Input: dimensioned drawing with shaded views. Units: mm. Origin: part minimum x, y, z. A direction names the side the tool comes from. Coordinates: 2 decimals unless noted, no trailing zeros. Write each loop counter-clockwise with the first axis right and the second up, starting at its lowest first coordinate (ties: lowest second). Pieces come first, ordered by that corner, then holes. Notation, with made-up numbers: (14, 38.5) -> (72, 38.5) arc R26 ccw to (72, 60.5) -> close; hole circle Ø5 at (26.5, 65). An arc over 180 degrees is marked (long way). One line per item, written item: value. Start each with the question number.
1. Section query B-B, the plane y = 13. Output: boundary loops of the cut face in (x, z) (1 decimal).
2. Access query for the marked faces 3 and 4. Directions: +Z, -Z, +X, -X, +Y, -Y. A direction counts if a zero-diameter tool reaches every point of the face in a straight line with its end or side. Return the directions, or none.
3. Line query: line 1 (Y direction, x = 0.95, z = 12.5); line 2 (Y direction, x = 0.25, z = 3.5) (1 decimal); line 3 (Z direction, x = 0.35, y = 10.5) (1 decimal). Output: solid intervals per line, ascending.
4. Section query D-D, the plane z = 7.75. Output: boundary loops of the cut face in (x, y).
5. Section query C-C, the plane y = 8.5. Output: boundary loops of the cut face in (x, z) (1 decimal).
6. First-contact query: P1, Ø0.5, axis at x = 0.5, y = 15.5, coming from the +Z side. Flat tip, straight axial feed; report the tip coordinate or a pass-through.
7. Mould query, pull axis Z, two halves, no side actions, for the marked faces 1 and 2. Classes: released by +Z, released by -Z, zero draft, split by the parting line, or undercut.
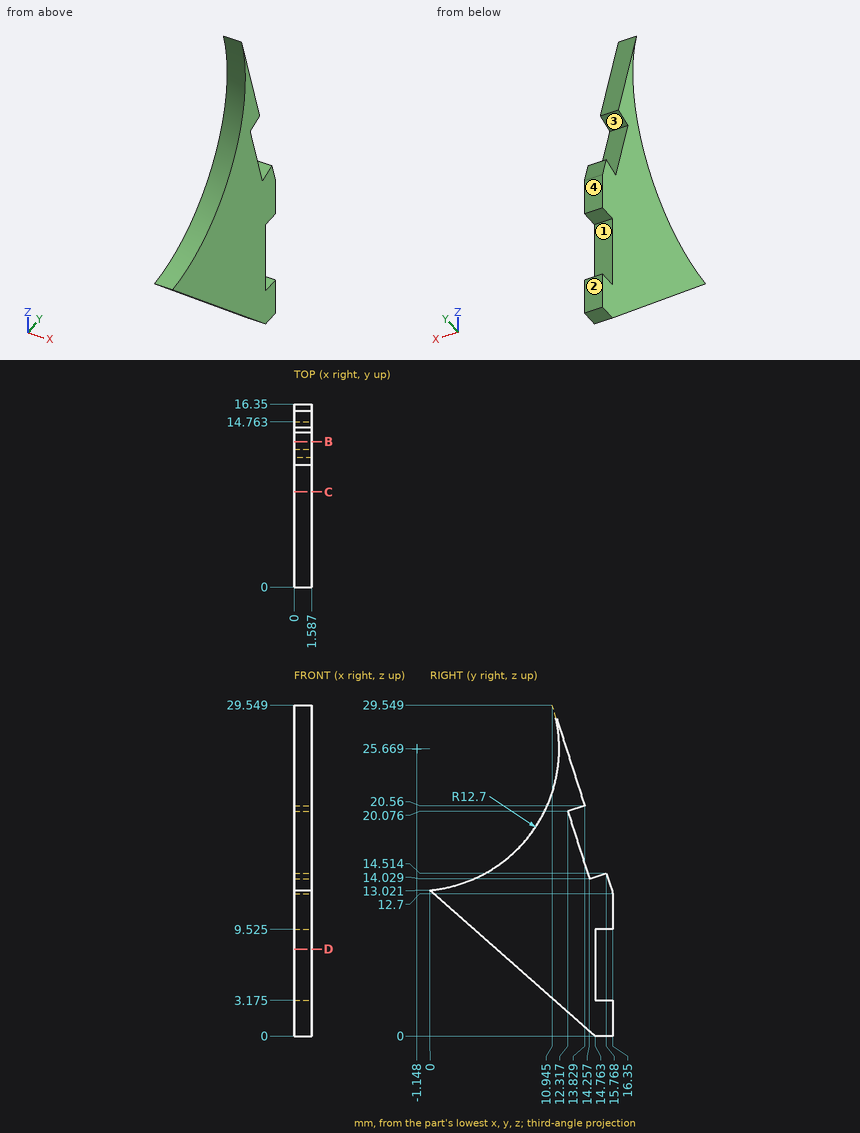
Computed values:
1. outline: (0, 1.6) -> (1.6, 1.6) -> (1.6, 17.9) -> (0, 17.9) -> close; (0, 20.3) -> (1.6, 20.3) -> (1.6, 23.1) -> (0, 23.1) -> close
2. face 3: +X, -X, +Y
2. face 4: +Z, -Z, +X, -X, +Y
3. line 1: y = 0.59 to 16.35
3. line 2: y = 10.8 to 14.8
3. line 3: z = 3.8 to 20.6
4. outline: (0, 5.98) -> (1.59, 5.98) -> (1.59, 14.76) -> (0, 14.76) -> close
5. outline: (0, 5.5) -> (1.6, 5.5) -> (1.6, 17.4) -> (0, 17.4) -> close
6. P1: stops at z = 14.51
7. face 1: undercut
7. face 2: zero draft
